Build history of the part. All positions in model axes, mm. Round coordinates to 2 decimals unless told otherwise and drop trailing zeros. Loops run counter-clockwise (first coordinate to the right, second up) from the corner with the lowest first, then second, coordinate; pieces in that order, holes last. Notation, with made-up numbers: (-33, 68) -> (-3, 68) arc R18 cw to (-3, 82) -> close; hole circle Ø6 at (4.5, 79.25). An arc over 180 degrees is marked (long way). Put each result on its own line as item: value. Start each with the question number.
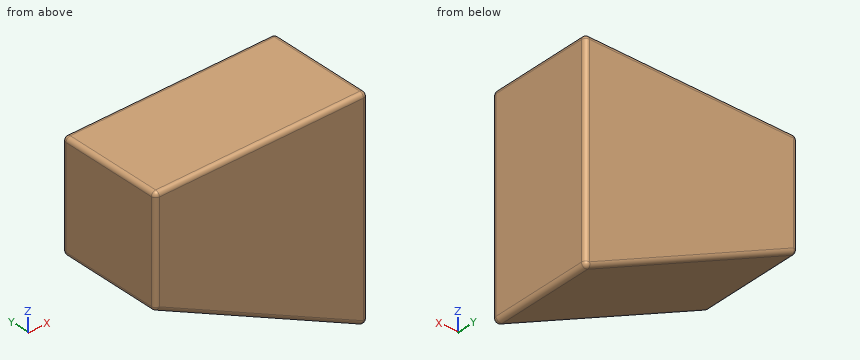
```python
from build123d import *

# Parameters (mm, degrees)
SKETCH1_W           = 10
SKETCH1_H           = 5
BOSS_EXTRUDE1_DEPTH = 5
FILLET1_R           = 0.2


with BuildPart() as part:
    # Sketch1 → Boss-Extrude1 (new body)
    with BuildSketch(Plane(origin=(0, 0, 0), x_dir=(1, 0, 0), z_dir=(0, 1, 0))):
        Polygon((10, 10), (10, 5), (0, 5), align=None)
        with Locations((5, 2.5)):
            Rectangle(SKETCH1_W, SKETCH1_H)
    extrude(amount=BOSS_EXTRUDE1_DEPTH)

    # Fillet1
    fillet1_edges = [part.edges().sort_by_distance(p)[0] for p in [
        (5, 5, -7.5),
        (0, 5, -2.5),
        (5, 5, 0),
        (10, 5, -5),
        (5, 0, 0),
        (0, 0, -2.5),
        (5, 0, -7.5),
        (10, 0, -5),
        (10, 2.5, 0),
        (0, 2.5, 0),
        (0, 2.5, -5),
        (10, 2.5, -10),
    ]]
    fillet(fillet1_edges, radius=FILLET1_R)


solid = part.part
```
Item 1: Drop a flat-ended pin along its axis: pin 1 (1.5 mm diameter, centred on y = 4.5, z = -8, fed in from -X). Give the stop position or say it passes through.
Item 2: Wall check: line 1 (X direction, y = 2.9, z = -7.5); line 2 (Z direction, x = 3.75, y = 0.7) (3 decimals); line 3 (X direction, y = 1.55, z = -9.25). Give the ranges that are in metal, low to high. Write a range as from..to.
Item 3: Cut at A-A on y = 1.3. Write the cut outline in (x, z).
Ans:
1. pin 1: stops at x = 4.5
2. line 1: x = 5..10
2. line 2: z = -6.875..0
2. line 3: x = 8.5..10
3. outline: (0, -4.88) arc R0.2 ccw to (0.11, -5.06) -> (9.71, -9.86) arc R0.2 ccw to (10, -9.68) -> (10, -0.2) arc R0.2 ccw to (9.8, 0) -> (0.2, 0) arc R0.2 ccw to (0, -0.2) -> close
